Input: part model. Units: mm. Frame: model coordinates. A direction names the side the tool comes from. Coordinates: 2 decimals unless noted, no trailing zeros. Loops run counter-clockwise (first coordinate to the right, second up) from the corner with the lowest first, then second, coordinate; pieces in that order, holes last. Notation, with made-up numbers: (65, -27.75) - (107, -27.75) arc R26 ccw to (107, -4.75) - close; hole circle Ø8 at (72, 63.5). An arc over 180 degrees is marked (long way). Use one line per item in the form item = value.
from build123d import *

# Parameters (mm, degrees)
SKETCH2_R          = 12.7
CUT_EXTRUDE1_DEPTH = 77.2
SKETCH3_R          = 76.2
CUT_EXTRUDE2_DEPTH = 23.876


with BuildPart() as part:
    # Sketch1 → Revolve1 (revolve)
    with BuildSketch(Plane(origin=(0, 0, 0), x_dir=(0, 0, -1), z_dir=(1, 0, 0))):
        with BuildLine():
            Line((0, 0), (0, 76.2))
            Line((0, 76.2), (-21.180812514, 76.2))
            ThreePointArc((-21.180812514, 76.2), (-37.345273532, 82.895538982), (-44.040812514, 99.06))
            Line((-44.040812514, 99.06), (-44.040812514, 104.14))
            ThreePointArc((-44.040812514, 104.14), (-50.736351496, 120.304461018), (-66.900812514, 127))
            Line((-66.900812514, 127), (-76.2, 127))
            Line((-76.2, 127), (-76.2, 0))
            Line((-76.2, 0), (0, 0))
        make_face()
    revolve(axis=Axis((0, 0, 0), (0, 1, 0)))

    # Sketch2 → Cut-Extrude1 (cut, through all)
    with BuildSketch(Plane(origin=(0, 76.2, 0), x_dir=(1, 0, 0), z_dir=(0, 1, 0))):
        Circle(SKETCH2_R)
    extrude(amount=-CUT_EXTRUDE1_DEPTH, mode=Mode.SUBTRACT)

    # Sketch3 → Cut-Extrude2 (cut)
    with BuildSketch(Plane(origin=(0, 0, 0), x_dir=(-1, 0, 0), z_dir=(0, -1, 0))):
        Circle(SKETCH3_R)
    extrude(amount=-CUT_EXTRUDE2_DEPTH, mode=Mode.SUBTRACT)


solid = part.part
Q1. Pull-direction query (X, two-part tool) for faces 3 (the cylindrical face through (22.89, 74.72, 72.68)), 4 (the cylindrical face through (-2.75, 50.4, 12.4)), 5 (the cylindrical face through (43.666, 101.636, -5.733)), 6 (the flat face through (1, 23.876, 16)); classes: pulls with the +X half, pulls with the -X half, needs draft (parallel to the pull), parting line crosses it, or undercut.
Check values:
face_3 = parting line crosses it
face_4 = undercut
face_5 = undercut
face_6 = needs draft
Q2. First-contact query: P1, Ø12, axis at y = 95, z = -23.5, coming from the -X side; P2, Ø5, axis at y = 68.5, z = -21.5, coming from the +X side; P3, Ø6, axis at y = 38, z = 13, coming from the +X side. Flat tips, straight axial feed; report the tip coordinate or a pass-through.
Check values:
P1 = -74.16
P2 = 73.79
P3 = 75.54
Q3. Cut plane A-A, the plane y = 62.5. Return loops of the section in (x, z), then the cut area to 3 significant figures.
Check values:
outline = circle Ø152.4 at (0, 0); hole circle Ø25.4 at (0, 0)
area = 17,700 mm²
Q4. Ray query, line 1 along X through (y, z) = (47, 0); line 2 along X through (y, z) = (102.2, 0). Return the intervals inside material, ascending. Write a range as [from, to].
Check values:
line_1 = [-76.2, -12.7], [12.7, 76.2]
line_2 = [-76.2, -44.04], [44.04, 76.2]
Q5. Cut plane B-B, the plane y = 113. Return loops of the section in (x, z).
Check values:
outline = circle Ø152.4 at (0, 0); hole circle Ø91.66 at (0, 0)
Q6. Set-up query: faces 1 (the flat face through (-67.4, 127, 0.4)), 2 (the flat face through (-9.1, 76.2, -9.1)). Return all of +Z, -Z, +X, -X, +Y, -Y with unobstructed straight access to the full face (end or side cutting, diameter ignored); none if empty.
Check values:
face_1 = +Z, -Z, +X, -X, +Y
face_2 = +Y
